The drawing under review shows one solid part. Ordinate dimensions are in mm from its lowest x, y, z. Coordinates: 2 decimals unless noted, no trailing zeros. Order: outer loops, then holes, each group sorted by start corner. A loop starts at its lowest first (then second) coordinate and runs counter-clockwise, first axis right, second up.
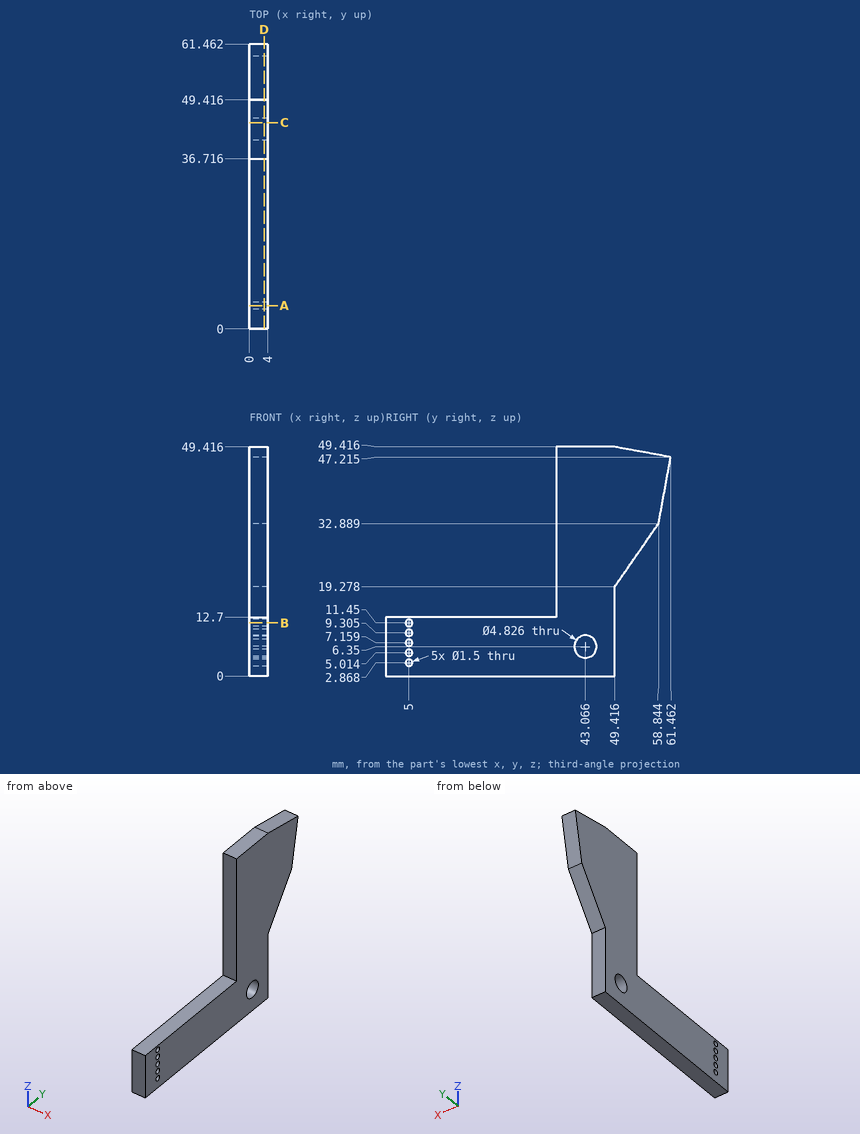
1. Take a section at D-D, the plane x = 3.2. Give the number of separate pieces and of enclosed holes in the cut face, plus the area to 3 significant figures.
Answer below:
separate pieces: 1
enclosed holes: 6
area: 1,300 mm2
2. Take a section at B-B, the plane z = 11.45. Give the boundary of the cut face in (x, y).
Answer below:
outline: (0, 0) - (4, 0) - (4, 4.25) - (0, 4.25) - close; (0, 5.75) - (4, 5.75) - (4, 49.42) - (0, 49.42) - close
3. Clearance check with flat-ended pins moving along their axes: pin 1 Ø2 at (x, y) = (2, 22) entering from +Z; pin 2 Ø2 at (x, z) = (2.5, 5.5) entering from +Y; pin 3 Ø10 at (y, z) = (24.5, 19) entering from -X; pin 4 Ø2 at (x, z) = (1, 23.5) entering from -Y. State where each tip first meets the part, or that it passes through.
Answer below:
pin 1: stops at z = 12.7
pin 2: stops at y = 49.42
pin 3: passes through
pin 4: stops at y = 36.72
4. Take a section at A-A, the plane y = 5. Give the boundary of the cut face in (x, z) (1 decimal).
Answer below:
outline: (0, 0) - (4, 0) - (4, 2.1) - (0, 2.1) - close; (0, 3.6) - (4, 3.6) - (4, 4.3) - (0, 4.3) - close; (0, 5.8) - (4, 5.8) - (4, 6.4) - (0, 6.4) - close; (0, 7.9) - (4, 7.9) - (4, 8.6) - (0, 8.6) - close; (0, 10.1) - (4, 10.1) - (4, 10.7) - (0, 10.7) - close; (0, 12.2) - (4, 12.2) - (4, 12.7) - (0, 12.7) - close
5. Take a section at C-C, the plane y = 44.5. Give the boundary of the cut face in (x, z), plus the area to 3 significant figures.
Answer below:
outline: (0, 0) - (4, 0) - (4, 4.41) - (0, 4.41) - close; (0, 8.29) - (4, 8.29) - (4, 49.42) - (0, 49.42) - close
area: 182 mm2
6. To check wall thickness, follow L1, parallel to Z at x = 1.3, y = 5 (1 decimal); L2, parallel to Y at x = 1.1, z = 6.35; L3, parallel to Y at x = 3.55, z = 4.5 (1 decimal). State the ranges of each line that lie inside material, in increasing order.
Answer below:
L1: z = 0 to 2.1, 3.6 to 4.3, 5.8 to 6.4, 7.9 to 8.6, 10.1 to 10.7, 12.2 to 12.7
L2: y = 0 to 40.65, 45.48 to 49.42
L3: y = 0 to 4.5, 5.5 to 41.5, 44.6 to 49.4
